from build123d import *

# Parameters (mm, degrees)
SKETCH3_W           = 5
SKETCH3_H           = 5
BOSS_EXTRUDE1_DEPTH = 37.5
SKETCH4_R           = 1.5
CUT_EXTRUDE1_DEPTH  = 5
SKETCH5_W           = 3.469365962
SKETCH5_H           = 1.189282553
BOSS_EXTRUDE2_DEPTH = 8
SKETCH6_W           = 20.090906928
SKETCH6_H           = 16.444349254
CUT_EXTRUDE2_DEPTH  = 10.5
FILLET5_R           = 1
FILLET6_R           = 1
FILLET7_R           = 1
FILLET8_R           = 1


with BuildPart() as part:
    # Sketch1 → Revolve1 (revolve)
    with BuildSketch(Plane.XY):
        with BuildLine():
            Line((-0.590277778, 15.201388889), (-0.590277778, -0.798611111))
            ThreePointArc((-0.590277778, -0.798611111), (7.409722222, 7.201388889), (-0.590277778, 15.201388889))
        make_face()
    revolve(axis=Axis((-0.590277778, 15.201388889, 0), (0, -1, 0)))

    # Sketch3 → Boss-Extrude1 (add)
    with BuildSketch(Plane(origin=(0, 0, 0), x_dir=(-1, 0, 0), z_dir=(0, 0, -1))):
        with Locations((0.590277778, 7.201388889)):
            Rectangle(SKETCH3_W, SKETCH3_H)
    extrude(amount=-BOSS_EXTRUDE1_DEPTH)

    # Sketch4 → Cut-Extrude1 (cut)
    with BuildSketch(Plane.XZ.offset(-4.701388889)):
        with Locations(Location((-0.590277778, 34.5, 0), (0, 0, 270))):
            Circle(SKETCH4_R)
    extrude(amount=-CUT_EXTRUDE1_DEPTH, mode=Mode.SUBTRACT)


with BuildPart() as body_2:
    # Sketch5 → Boss-Extrude2 (new body)
    with BuildSketch(Plane(origin=(0, 0, 0), x_dir=(1, 0, 0), z_dir=(0, 1, 0))):
        with Locations((0, 12.70312089)):
            Rectangle(SKETCH5_W, SKETCH5_H)
    extrude(amount=BOSS_EXTRUDE2_DEPTH)


with BuildPart() as cut_extrude2_tool:
    # Sketch6 → Cut-Extrude2 (new body)
    with BuildSketch(Plane(origin=(0, 0, -13.297762167), x_dir=(-1, 0, 0), z_dir=(0, 0, -1))):
        with Locations((0.125748138, 7.050416756)):
            Rectangle(SKETCH6_W, SKETCH6_H)
    extrude(amount=-CUT_EXTRUDE2_DEPTH)


with BuildPart() as part_1:
    add(part.part)

    # Cut-Extrude2: cut by cut_extrude2_tool
    add(cut_extrude2_tool.part, mode=Mode.SUBTRACT)

    # Fillet5
    fillet5_edges = [part_1.edges().sort_by_distance(p)[0] for p in [
        (-3.090277778, 9.701388889, 22.338175024),
    ]]
    fillet(fillet5_edges, radius=FILLET5_R - 0.0001)  # a hair under: the kernel refuses the full size

    # Fillet6
    fillet6_edges = [part_1.edges().sort_by_distance(p)[0] for p in [
        (1.909722222, 9.701388889, 22.338175024),
    ]]
    fillet(fillet6_edges, radius=FILLET6_R)

    # Fillet7
    fillet7_edges = [part_1.edges().sort_by_distance(p)[0] for p in [
        (1.909722222, 4.701388889, 22.338175024),
    ]]
    fillet(fillet7_edges, radius=FILLET7_R)

    # Fillet8
    fillet8_edges = [part_1.edges().sort_by_distance(p)[0] for p in [
        (-3.090277778, 4.701388889, 22.338175024),
    ]]
    fillet(fillet8_edges, radius=FILLET8_R - 0.0001)  # a hair under: the kernel refuses the full size


with BuildPart() as body_2_1:
    add(body_2.part)

    # Cut-Extrude2: cut by cut_extrude2_tool
    add(cut_extrude2_tool.part, mode=Mode.SUBTRACT)


solid = part_1.part
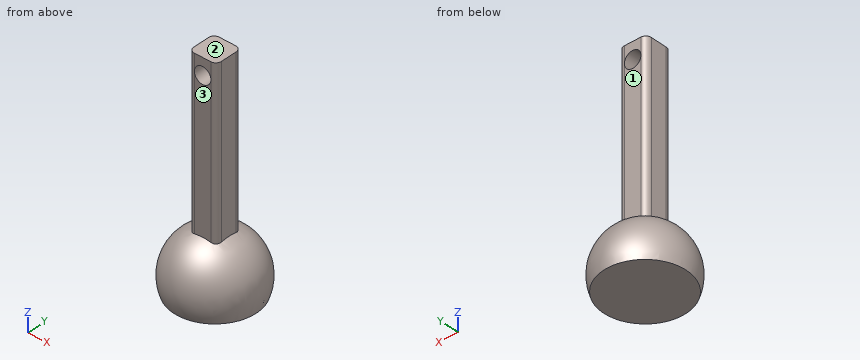
CAD build for the part. Positions are in the model's coordinates, mm. Face numbers are marked on the shaded views. A direction names the side the tool comes from. Give positions to 0.01 mm unless a question says otherwise; leave off trailing zeros. Loops run counter-clockwise (first coordinate to the right, second up) from the corner with the lowest first, then second, coordinate; pieces in that order, holes last. Notation, with made-up numbers: M -9,-37.5 L -2,-37.5 A22 cw -2,-11.5 Z; hole C 4.5,82 d3. An arc over 180 degrees is marked long. Answer in a Markdown table with one row per item. Add a question column.
Item 1: Band-saw the part on B-B on y = 7.25. Give the cut face in (x, z), then the cut area to 3 significant figures.
Item 2: Band-saw the part on A-A on z = 34. Give the cut face in (x, y).
Item 3: Band-saw the part on D-D on x = -7.25. Give the cut face in (y, z).
Item 4: Band-saw the part on C-C on z = 26. Give the cut face in (x, y).
Item 5: Drop flat-ended pins along their axis: P1, Ø3, axis at y = 11.5, z = 6, coming from the +X side; P2, Ø5, axis at x = 2.5, z = 20.5, coming from the +Y side; P3, Ø3, axis at x = -0.5, z = 25, coming from the -Y side. Give the stop position or say it passes through.
Item 6: Tool access for the marked faces 1, 2 and 3: list every direction of +Z, -Z, +X, -X, +Y, -Y with a clear straight run to the whole face (end or side of a thin tool).
Item 7: Probe probe 1 along X at (y, z) = (8.35, 34.5); probe 2 along Y at (x, z) = (-1, 20); probe 3 along X at (y, z) = (6.5, 21). List the from-to ranges inside material, lowest first.
Reply:
| question | item | result |
|---|---|---|
| 1 | outline | M -8.08,-2.8 L 6.9,-2.8 A8 ccw 1.91,7.6 L 1.91,37.5 L -3.09,37.5 L -3.09,7.6 A8 ccw Z; hole C -0.59,34.5 d3 |
| 1 | area | 285 mm^2 |
| 2 | outline | M -3.09,5.7 A1 ccw -2.09,4.7 L -2,4.7 L -2,9.7 L -2.09,9.7 A1 ccw -3.09,8.7 Z; M 0.82,4.7 L 0.91,4.7 A1 ccw 1.91,5.7 L 1.91,8.7 A1 ccw 0.91,9.7 L 0.82,9.7 Z |
| 3 | outline | M 3.76,-2.8 L 10.64,-2.8 A4.43 ccw long Z |
| 4 | outline | M -3.09,5.7 A1 ccw -2.09,4.7 L 0.91,4.7 A1 ccw 1.91,5.7 L 1.91,8.7 A1 ccw 0.91,9.7 L -2.09,9.7 A1 ccw -3.09,8.7 Z |
| 5 | P1 | stops at x = 4.83 |
| 5 | P2 | stops at y = 9.7 |
| 5 | P3 | stops at y = 4.7 |
| 6 | face 1 | +Z, +X, -X, +Y |
| 6 | face 2 | +Z, +X, -X, +Y, -Y |
| 6 | face 3 | +Z, +X, -X, -Y |
| 7 | probe 1 | x = -3.09 to -2.09, 0.91 to 1.91 |
| 7 | probe 2 | y = 4.7 to 9.7 |
| 7 | probe 3 | x = -3.09 to 1.91 |
